```python
from build123d import *

# Parameters (mm, degrees)
SKETCH1_W           = 150
SKETCH1_H           = 45
BOSS_EXTRUDE1_DEPTH = 5
SKETCH2_W           = 5
SKETCH2_H           = 45
BOSS_EXTRUDE2_DEPTH = 20
SKETCH3_W           = 5
SKETCH3_H           = 45
BOSS_EXTRUDE3_DEPTH = 20
SKETCH4_W           = 35
SKETCH4_H           = 11.8
CUT_EXTRUDE1_DEPTH  = 81.816149376
SKETCH5_W           = 30
SKETCH5_H           = 3
BOSS_EXTRUDE4_DEPTH = 4
SKETCH7_W           = 5
SKETCH7_H           = 45
BOSS_EXTRUDE5_DEPTH = 30
SKETCH8_W           = 79
SKETCH8_H           = 45
BOSS_EXTRUDE6_DEPTH = 32
CUT_EXTRUDE2_REACH  = 158.126
SKETCH9_R           = 14
FILLET1_R           = 10
SKETCH10_W          = 45
SKETCH10_H          = 5
BOSS_EXTRUDE7_DEPTH = 10
CUT_EXTRUDE3_REACH  = 88.604
SKETCH11_R          = 2.55
CUT_EXTRUDE4_DEPTH  = 4
LPATTERN1_COUNT     = 2
LPATTERN1_PITCH     = 30


with BuildPart() as part:
    # Sketch1 → Boss-Extrude1 (new body)
    with BuildSketch(Plane(origin=(0, 0, 0), x_dir=(1, 0, 0), z_dir=(0, 1, 0))):
        Rectangle(SKETCH1_W, SKETCH1_H)
    extrude(amount=BOSS_EXTRUDE1_DEPTH)

    # Sketch2 → Boss-Extrude2 (add)
    with BuildSketch(Plane.XZ):
        with Locations((72.5, 0)):
            Rectangle(SKETCH2_W, SKETCH2_H)
    extrude(amount=BOSS_EXTRUDE2_DEPTH)

    # Sketch3 → Boss-Extrude3 (add)
    with BuildSketch(Plane.XZ):
        with Locations((-9.5, 0)):
            Rectangle(SKETCH3_W, SKETCH3_H)
    extrude(amount=BOSS_EXTRUDE3_DEPTH)

    # Sketch4 → Cut-Extrude1 (cut, through all)
    with BuildSketch(Plane.XZ):
        with Locations((31.5, 0)):
            Rectangle(SKETCH4_W, SKETCH4_H)
    extrude(amount=-CUT_EXTRUDE1_DEPTH, mode=Mode.SUBTRACT)

    # Sketch5 → Boss-Extrude4 (add)
    with BuildSketch(Plane.XZ):
        with Locations((31.5, -7.4)):
            Rectangle(SKETCH5_W, SKETCH5_H)
    boss_extrude4 = extrude(amount=BOSS_EXTRUDE4_DEPTH)

    # Mirror1: Boss-Extrude4 across plane
    add(boss_extrude4.mirror(Plane.XY))

    # Sketch7 → Boss-Extrude5 (add)
    with BuildSketch(Plane(origin=(0, 5, 0), x_dir=(1, 0, 0), z_dir=(0, 1, 0))):
        with Locations((51.5, 0)):
            Rectangle(SKETCH7_W, SKETCH7_H)
    extrude(amount=BOSS_EXTRUDE5_DEPTH)

    # Sketch8 → Boss-Extrude6 (add)
    with BuildSketch(Plane(origin=(0, 5, 0), x_dir=(1, 0, 0), z_dir=(0, 1, 0))):
        with Locations((-35.5, 0)):
            Rectangle(SKETCH8_W, SKETCH8_H)
    extrude(amount=BOSS_EXTRUDE6_DEPTH)

    # Sketch9 → Cut-Extrude2 (cut, up to next)
    with BuildSketch(Plane.ZY.offset(75), mode=Mode.PRIVATE) as cut_extrude2_sk1:
        with Locations((0, 20)):
            Circle(SKETCH9_R)
    cut_extrude2_tool1 = extrude(cut_extrude2_sk1.sketch, amount=-CUT_EXTRUDE2_REACH, mode=Mode.PRIVATE) & part.part
    add(cut_extrude2_tool1.solids().sort_by_distance((-75, 20, 0))[0], mode=Mode.SUBTRACT)

    # Fillet1
    fillet1_edges = [part.edges().sort_by_distance(p)[0] for p in [
        (-35.5, 37, 22.5),
        (-35.5, 37, -22.5),
    ]]
    fillet(fillet1_edges, radius=FILLET1_R)

    # Sketch10 → Boss-Extrude7 (add)
    with BuildSketch(Plane.ZY.offset(-49)):
        with Locations((0, 29.5)):
            Rectangle(SKETCH10_W, SKETCH10_H)
    extrude(amount=BOSS_EXTRUDE7_DEPTH)

    # Sketch11 → Cut-Extrude3 (cut, up to next)
    with BuildSketch(Plane.XZ, mode=Mode.PRIVATE) as cut_extrude3_sk1:
        with Locations(Location((-60, 0, 0), (0, 0, 270))):
            Circle(SKETCH11_R)
    cut_extrude3_tool1 = extrude(cut_extrude3_sk1.sketch, amount=-CUT_EXTRUDE3_REACH, mode=Mode.PRIVATE) & part.part
    cut_extrude3 = cut_extrude3_tool1.solids().sort_by_distance((-60, 0, 0))[0]
    add(cut_extrude3, mode=Mode.SUBTRACT)

    # Sketch12 → Cut-Extrude4 (cut)
    with BuildSketch(Plane.XZ):
        Polygon((-55.95, -2.33826859), (-55.95, 2.33826859), (-60, 4.67653718), (-64.05, 2.33826859), (-64.05, -2.33826859), (-60, -4.67653718), align=None)
    cut_extrude4 = extrude(amount=-CUT_EXTRUDE4_DEPTH, mode=Mode.SUBTRACT)

    # LPattern1: Cut-Extrude3, Cut-Extrude4 ×2
    with Locations(*[(i * LPATTERN1_PITCH, 0, 0) for i in range(1, LPATTERN1_COUNT)]):
        add(cut_extrude3, mode=Mode.SUBTRACT)
        add(cut_extrude4, mode=Mode.SUBTRACT)


solid = part.part
```
For this review, take the finished solid that the model builds, in its own axes (mm). A direction names the side the tool comes from. Round coordinates to 2 decimals unless told otherwise and drop trailing zeros. Write each loop counter-clockwise with the first axis right and the second up, starting at its lowest first coordinate (ties: lowest second). Pieces come first, ordered by that corner, then holes. Notation, with made-up numbers: (-21.5, 4) - (0.5, 4) arc R37 cw to (0.5, 41) - close; hole circle Ø3 at (82, 36.5). An arc over 180 degrees is marked (long way). Use CSV: the item, a comma, the result in double quotes.
1) Add section C-C on z = 0. Count the separate pieces of the cut face and the enclosed holes in it, and give its area (3 significant figures).
Conclusion:
separate pieces,"5"
enclosed holes,"0"
area,"1,210 mm^2"
2) Wall thickness on line 1 along Z through (x, y) = (-60, 5.3); line 2 along X through (y, z) = (21.5, -19); line 3 along X through (y, z) = (-17, -17): over which ranges is each line inside the solid? List them lowest first. Write a range as from..to.
Conclusion:
line 1,"z = -22.5..-2.55, 2.55..22.5"
line 2,"x = -75..4, 49..54"
line 3,"x = -12..-7, 70..75"
3) The part is to be moulded in two halves that separate along Z. For faces 5 (the cylindrical face through (-34.95, 34.15, -19.49)), 6 (the cylindrical face through (-36.1, 7.6, 6.5)), 7 (the flat face through (31, -4, 7)), 8 (the flat face through (-62.053, 1.972, -3.491)), say which applies: pulls with the +Z half, pulls with the -Z half, needs draft (parallel to the pull), parting line crosses it, or undercut.
Conclusion:
face 5,"pulls with the -Z half"
face 6,"undercut"
face 7,"needs draft"
face 8,"undercut"
4) For faces 1 (the flat face through (-44, 0, 0)), 2 (the flat face through (46.5, -2, 7)), 3 (the flat face through (31, -2, -8.9)), 4 (the flat face through (31, 0, -5.9)), list the 3-axis set-ups (+Z, -Z, +X, -X, +Y, -Y) from which the entire face can be reached by the end or side of a thin tool; tool diameter is ignored.
Conclusion:
face 1,"+Z, -Z, -X, -Y"
face 2,"+Z, -Z, -Y"
face 3,"-Z, -Y"
face 4,"-Y"
5) Clearance check with flat-ended pins moving along their axes: pin 1 Ø3 at (x, z) = (42, -11) entering from -Y; pin 2 Ø2.5 at (x, z) = (-60, -0.5) entering from -Y; pin 3 Ø3 at (x, y) = (30.5, -3) entering from +Z; pin 4 Ø10 at (y, z) = (5.5, -9.5) entering from +X. State where each tip first meets the part, or that it passes through.
Conclusion:
pin 1,"stops at y = 0"
pin 2,"stops at y = 33.89"
pin 3,"stops at z = 8.9"
pin 4,"stops at x = 75"
6) Add section B-B on y = -14. Write out the cut boundary in (x, z), and give its area (3 significant figures).
Conclusion:
outline,"(-12, -22.5) - (-7, -22.5) - (-7, 22.5) - (-12, 22.5) - close; (70, -22.5) - (75, -22.5) - (75, 22.5) - (70, 22.5) - close"
area,"450 mm^2"
7) Add section A-A on y = 20. Write out the cut boundary in (x, z), and give its area (3 significant figures).
Conclusion:
outline,"(-75, -22.5) - (4, -22.5) - (4, -14) - (-75, -14) - close; (-75, 14) - (4, 14) - (4, 22.5) - (-75, 22.5) - close; (49, -22.5) - (54, -22.5) - (54, 22.5) - (49, 22.5) - close"
area,"1,570 mm^2"
8) Add section D-D on z = -15.5. Write out the cut boundary in (x, y), and give its area (3 significant figures).
Conclusion:
outline,"(-75, 0) - (-12, 0) - (-12, -20) - (-7, -20) - (-7, 0) - (70, 0) - (70, -20) - (75, -20) - (75, 5) - (54, 5) - (54, 35) - (49, 35) - (49, 32) - (39, 32) - (39, 27) - (49, 27) - (49, 5) - (4, 5) - (4, 36.54) - (-75, 36.54) - close"
area,"3,640 mm^2"
